Design review of the part built by this model. Coordinates are the model's own, in mm. A direction names the side the tool comes from. Coordinates: 2 decimals unless noted, no trailing zeros. Write each loop counter-clockwise with the first axis right and the second up, starting at its lowest first coordinate (ties: lowest second). Pieces come first, ordered by that corner, then holes. Notation, with made-up numbers: (44, 81.25) - (88, 81.25) arc R38 ccw to (88, 119.25) - close; hole circle Ø11 at (74, 44). An arc over 180 degrees is marked (long way). One line per item, written item: value.
from build123d import *

# Parameters (mm, degrees)
SKETCH1_W                = 55.88
SKETCH1_H                = 99.06
BOSS_EXTRUDE1_DEPTH      = 3.81
SKETCH2_W                = 55.88
SKETCH2_H                = 45.72
BOSS_EXTRUDE2_DEPTH      = 20.32
SKETCH3_W                = 55.88
SKETCH3_H                = 2.54
BOSS_EXTRUDE3_DEPTH      = 55.88
SKETCH4_W                = 11.43
SKETCH4_H                = 55.911789182
SKETCH4_W_2              = 55.88
BOSS_EXTRUDE4_DEPTH      = 10.16
BOSS_EXTRUDE4_DEPTH_BACK = 2.54


with BuildPart() as part:
    # Sketch1 → Boss-Extrude1 (new body)
    with BuildSketch(Plane.XY):
        Rectangle(SKETCH1_W, SKETCH1_H)
    extrude(amount=BOSS_EXTRUDE1_DEPTH)

    # Sketch2 → Boss-Extrude2 (add)
    with BuildSketch(Plane.XY.offset(3.81)):
        with Locations((0, 26.67)):
            Rectangle(SKETCH2_W, SKETCH2_H)
    extrude(amount=BOSS_EXTRUDE2_DEPTH)

    # Sketch3 → Boss-Extrude3 (add)
    with BuildSketch(Plane.XZ.offset(-3.81)):
        with Locations((0, 22.86)):
            Rectangle(SKETCH3_W, SKETCH3_H)
    extrude(amount=BOSS_EXTRUDE3_DEPTH)

    # Sketch4 → Boss-Extrude4 (add, two sides)
    with BuildSketch(Plane.XY.offset(24.13)) as boss_extrude4_sk:
        with Locations((-33.655, -24.114105409)):
            Rectangle(SKETCH4_W, SKETCH4_H)
        with Locations((0, -24.114105409)):
            Rectangle(SKETCH4_W_2, SKETCH4_H)
        with Locations((33.655, -24.114105409)):
            Rectangle(SKETCH4_W, SKETCH4_H)
    extrude(amount=BOSS_EXTRUDE4_DEPTH)
    extrude(boss_extrude4_sk.sketch, amount=-BOSS_EXTRUDE4_DEPTH_BACK)


solid = part.part
1. Consider section D-D, the plane z = 12. Write out the cut boundary in (x, y).
Answer block:
outline: (-27.94, 3.81) - (27.94, 3.81) - (27.94, 49.53) - (-27.94, 49.53) - close
2. Mouldability with a two-part tool opening along Z and no side actions: class faces 4 (the face through (0, 27, 24.13)), 5 (the face through (-1, -24, 21.59)), 6 (the face through (0, 3.81, 13)), 7 (the face through (0, 49.53, 12)) as released by +Z, released by -Z, zero draft, split by the parting line, or undercut.
Answer block:
face 4: released by +Z
face 5: undercut
face 6: undercut
face 7: zero draft
3. Consider section C-C, the plane y = 39. Write out the cut boundary in (x, z).
Answer block:
outline: (-27.94, 0) - (27.94, 0) - (27.94, 24.13) - (-27.94, 24.13) - close
4. Wall thickness on line 1 along Z through (x, y) = (-24.5, -46); line 2 along Z through (x, y) = (-30, -21); line 3 along Y through (x, z) = (7, 25.5): over which ranges is each line inside the solid? List them lowest first.
Answer block:
line 1: z = 0 to 3.81, 21.59 to 34.29
line 2: z = 21.59 to 34.29
line 3: y = -52.07 to 3.84
5. Insertion check: pin 1 Ø6 at (y, z) = (-26, 4) entering from -X; pin 2 Ø3 at (x, z) = (29, 13) entering from +Y; pin 3 Ø1.9 at (x, z) = (0, 2) entering from -Y; pin 4 Ø12 at (y, z) = (16, 9.5) entering from +X. Each pin has a flat end and moves straight along its axis. Give the tip position at first contact, or say it passes through.
Answer block:
pin 1: stops at x = -27.94
pin 2: stops at y = 49.53
pin 3: stops at y = -49.53
pin 4: stops at x = 27.94
6. Consider section A-A, the plane y = -3. Write out the cut boundary in (x, z), then the cut area to 3 significant figures.
Answer block:
outline: (-39.37, 21.59) - (39.37, 21.59) - (39.37, 34.29) - (-39.37, 34.29) - close; (-27.94, 0) - (27.94, 0) - (27.94, 3.81) - (-27.94, 3.81) - close
area: 1,210 mm^2
7. Consider section B-B, the plane x = -1. Write out the cut boundary in (y, z).
Answer block:
outline: (-52.07, 21.59) - (3.81, 21.59) - (3.81, 3.81) - (-49.53, 3.81) - (-49.53, 0) - (49.53, 0) - (49.53, 24.13) - (3.84, 24.13) - (3.84, 34.29) - (-52.07, 34.29) - close
8. For faces 1 (the face through (0, 1, 0)), 2 (the face through (0, -22, 3.81)), 3 (the face through (0, -49.53, 2)), list the 3-axis set-ups (+Z, -Z, +X, -X, +Y, -Y) from which the entire face can be reached by the end or side of a thin tool; tool diameter is ignored.
Answer block:
face 1: -Z, +X, -X, +Y, -Y
face 2: +X, -X, -Y
face 3: -Z, +X, -X, -Y
